from build123d import *

# Parameters (mm, degrees)
SKETCH1_R           = 7
BOSS_EXTRUDE2_DEPTH = 30
BOSS_EXTRUDE4_DEPTH = 6
RIB3_REACH          = 55.749
SKETCH5_WALL_W      = 157.872383692
SKETCH5_WALL_H      = 7


with BuildPart() as part:
    # Sketch1 → Boss-Extrude2 (new body)
    with BuildSketch(Plane(origin=(0, 0, 0), x_dir=(1, 0, 0), z_dir=(0, 1, 0))):
        with BuildLine():
            Line((0, 0), (30, 0))
            Line((30, 0), (30, 18))
            ThreePointArc((30, 18), (15, 33), (0, 18))
            Line((0, 18), (0, 0))
        make_face()
        with Locations(Location((15, 18, 0), (0, 0, 270))):
            Circle(SKETCH1_R, mode=Mode.SUBTRACT)
    extrude(amount=BOSS_EXTRUDE2_DEPTH)

    # Sketch3 → Boss-Extrude4 (add)
    with BuildSketch(Plane(origin=(0, 0, 0), x_dir=(-1, 0, 0), z_dir=(0, -1, 0))):
        Polygon((-21, -42), (-30, -33), (-30, 0), (0, 0), (0, -33), (-9, -42), align=None)
    extrude(amount=-BOSS_EXTRUDE4_DEPTH)

    # Sketch5 wall → Rib3 (add, up to next)
    with BuildSketch(Plane(origin=(15, 18, 21), x_dir=(0, -0.496138938357, 0.868243142124), z_dir=(0, 0.868243142124, 0.496138938357)), mode=Mode.PRIVATE) as rib3_sk1:
        Rectangle(SKETCH5_WALL_W, SKETCH5_WALL_H)
    rib3_tool1 = extrude(rib3_sk1.sketch, amount=-RIB3_REACH, mode=Mode.PRIVATE) - part.part
    add(rib3_tool1.solids().sort_by_distance((15, 18, 21))[0])


solid = part.part
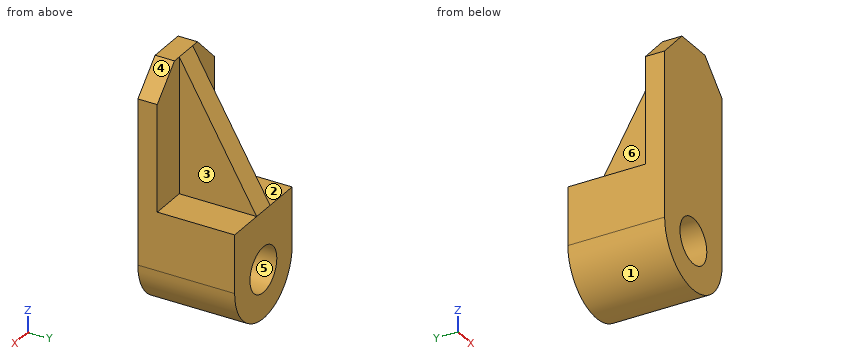
The listing builds one solid part. Answer for the finished solid, in the listing's coordinates (mm). Face numbers are marked on the shaded views. A direction names the side the tool comes from. Give positions to 0.01 mm unless a question says otherwise; leave off trailing zeros. Order: outer loops, then holes, each group sorted by start corner. A loop starts at its lowest first (then second) coordinate and runs counter-clockwise, first axis right, second up. Notation, with made-up numbers: (61, -38.75) -> (113, -38.75) arc R33 ccw to (113, -8.75) -> close; hole circle Ø4 at (-33, 76). An arc over 180 degrees is marked (long way). Put each result on its own line as item: value.
Item 1: A cutting plane is placed at C-C on z = 8. Give the vertices of the cut face in (x, y).
Established:
outline: (0, 0) -> (30, 0) -> (30, 6) -> (18.5, 6) -> (18.5, 25.43) -> (11.5, 25.43) -> (11.5, 6) -> (0, 6) -> close
Item 2: A cutting plane is placed at D-D on z = -17. Give the vertices of the cut face in (x, y).
Established:
outline: (0, 0) -> (8.07, 0) -> (8.07, 30) -> (0, 30) -> close; (21.93, 0) -> (30, 0) -> (30, 30) -> (21.93, 30) -> close
Item 3: A cutting plane is placed at B-B on y = 11. Give the vertices of the cut face in (x, z), plus the area to 3 significant figures.
Established:
outline: (0, -18) arc R15 ccw to (30, -18) -> (30, 0) -> (18.5, 0) -> (18.5, 33.25) -> (11.5, 33.25) -> (11.5, 0) -> (0, 0) -> close; hole circle Ø14 at (15, -18)
area: 972 mm^2
Item 4: For a pull along Z with two mould halves and no side action, classify the marked faces 4, 5 and 6 as released by +Z, released by -Z, zero draft, split by the parting line, or undercut.
Established:
face 4: released by +Z
face 5: undercut
face 6: zero draft
Item 5: Straight lines are drawn through the part: line 1 (X direction, y = 15.25, z = -18); line 2 (Y direction, x = 9.75, z = 13); line 3 (X direction, y = 6.5, z = 34.5). For each, find the intervals that lie inside material, in ascending order.
Established:
line 1: x = 0 to 8, 22 to 30
line 2: y = 0 to 6
line 3: x = 11.5 to 18.5
Item 6: Given P1, Ø6, axis at x = 4.5, y = 21, coming from the +Z side; P2, Ø12, axis at x = 23, y = 23.5, coming from the -Z side; P3, Ø4, axis at x = 27, y = 16, coming from the -Z side; P4, Ø12.5, axis at x = 15, z = -18, coming from the -Y side, each flat-ended and moving along its own axis, determine where each tip first touches the part or whether it passes through.
Established:
P1: stops at z = 0
P2: stops at z = -32.87
P3: stops at z = -29.18
P4: passes through
Item 7: For the marked faces 1, 2 and 3, determine the directions among +Z, -Z, +X, -X, +Y, -Y from which every point of the face is accessible in a straight line to the end or side of a thin tool.
Established:
face 1: -Z, +Y, -Y
face 2: +Z, -X, +Y
face 3: +Z, +X, +Y
Item 8: A cutting plane is placed at A-A on x = 15. Give the vertices of the cut face in (y, z).
Established:
outline: (0, -33) -> (30, -33) -> (30, -25) -> (0, -25) -> close; (0, -11) -> (30, -11) -> (30, 0) -> (6, 42) -> (0, 42) -> close
